Part print with two shaded views. Sizes in mm from the minimum x, y, z corner. Coordinates: 2 decimals unless noted, no trailing zeros. Write each loop counter-clockwise with the first axis right and the second up, starting at its lowest first coordinate (ties: lowest second). Pieces come first, ordered by that corner, then holes. Notation, with made-up numbers: (-16.75, 15.5) - (12.25, 15.5) arc R21 ccw to (12.25, 38.5) - close; hole circle Ø2 at (7.25, -7). An arc over 180 degrees is marked (long way). Answer in a Markdown table with one row per item. Add a question column.
Q1. Band-saw the part on D-D (x = 11). List the corners of the cut face in (y, z).
Q2. Two-plate mould, pull along X, no slides. Class the marked faces 1, 2 and 3: +X half, -X half, draft (parallel to the pull), parting line (faces both ways), or undercut.
Q3. Band-saw the part on A-A (y = 7). List the corners of the cut face in (x, z).
Q4. Band-saw the part on B-B (z = 2). List the corners of the cut face in (x, y).
Q5. Pin check, flat tips, straight feed: pin 1 (1.9 mm diameter, centred on x = 13.5, z = 53, fed in from -Y); pin 2 (0.7 mm diameter, centred on x = 1, y = 3, fed in from +Z); pin 3 (5 mm diameter, centred on x = 26, z = 49.8, fed in from -Y); pin 4 (2.5 mm diameter, centred on x = 26, z = 2, fed in from +Y). Stop position of each tip, or through.
Q6. Band-saw the part on C-C (y = 12). List the corners of the cut face in (x, z), and give its area (3 significant figures).
Q7. Drill centre lines: line 1 along X through (y, z) = (10.7, 49.8); line 2 along X through (y, z) = (12.25, 17); line 3 along X through (y, z) = (9.5, 14). Where is each one in solid material? Low to high. Write a range as from..to.
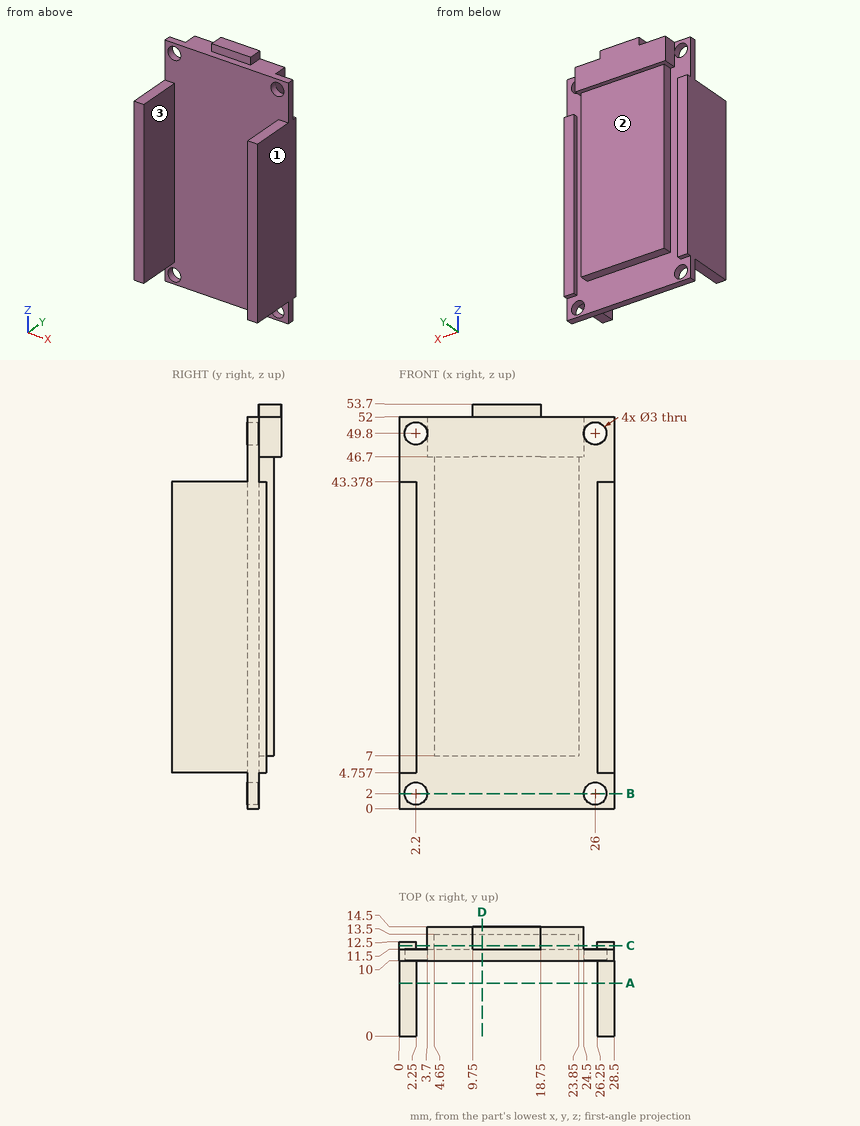
Checked values:
| question | item | result |
|---|---|---|
| 1 | outline | (10, 0) - (11.5, 0) - (11.5, 7) - (13.5, 7) - (13.5, 46.7) - (14.5, 46.7) - (14.5, 53.7) - (11.5, 53.7) - (11.5, 52) - (10, 52) - close |
| 2 | face 1 | +X half |
| 2 | face 2 | draft |
| 2 | face 3 | undercut |
| 3 | outline | (0, 4.76) - (2.25, 4.76) - (2.25, 43.38) - (0, 43.38) - close; (26.25, 4.76) - (28.5, 4.76) - (28.5, 43.38) - (26.25, 43.38) - close |
| 4 | outline | (0, 10) - (0.7, 10) - (0.7, 11.5) - (0, 11.5) - close; (3.7, 10) - (24.5, 10) - (24.5, 11.5) - (3.7, 11.5) - close; (27.5, 10) - (28.5, 10) - (28.5, 11.5) - (27.5, 11.5) - close |
| 5 | pin 1 | stops at y = 11.5 |
| 5 | pin 2 | stops at z = 43.38 |
| 5 | pin 3 | stops at y = 10 |
| 5 | pin 4 | passes through |
| 6 | outline | (0, 4.76) - (2.25, 4.76) - (2.25, 43.38) - (0, 43.38) - close; (3.7, 46.7) - (4.65, 46.7) - (4.65, 7) - (23.85, 7) - (23.85, 46.7) - (24.5, 46.7) - (24.5, 52) - (18.75, 52) - (18.75, 53.7) - (9.75, 53.7) - (9.75, 52) - (3.7, 52) - close; (26.25, 4.76) - (28.5, 4.76) - (28.5, 43.38) - (26.25, 43.38) - close |
| 6 | area | 1,060 mm² |
| 7 | line 1 | x = 0..0.7, 3.7..24.5, 27.5..28.5 |
| 7 | line 2 | x = 0..2.25, 4.65..23.85, 26.25..28.5 |
| 7 | line 3 | x = 0..2.25, 26.25..28.5 |
